Check sheet for the drawn part. Datum: minimum x, y, z corner. Units: mm. A direction names the side the tool comes from. Coordinates: 2 decimals unless noted, no trailing zeros. Write each loop counter-clockwise with the first axis right and the second up, starting at its lowest first coordinate (ties: lowest second). Pieces come first, ordered by that corner, then holes. Notation, with made-up numbers: M -9.75,65.5 L 9.25,65.5 A22 ccw 9.25,85.5 Z; hole C -17.75,-21.5 d1. An arc over 180 degrees is marked long. Answer as CSV lines item,"result". Start each with the question number.
Q1. Thickness scan on line 1 along Y through (x, z) = (11, 17.25) (3 decimals); line 2 along Z through (x, y) = (8.25, 4); line 3 along Z through (x, y) = (6.5, 9.5) (1 decimal). Record the ranges inside material, lowest first. Write a range as from..to.
Q2. Sectioned sample at B-B, the plane x = 6.5. Record the cut outline in (y, z) (1 decimal).
Q3. Sectioned sample at C-C, the plane z = 3.5. Record the cut outline in (x, y) (3 decimals).
Q4. Sectioned sample at D-D, the plane x = 3.5. Record the cut outline in (y, z) (3 decimals).
Q5. Sectioned sample at A-A, the plane y = 1.5. Record the cut outline in (x, z), then the cut area to 3 significant figures.
Q6. Access from +Z, -Z, +X, -X, +Y, -Y to the whole of each face (thin tool, end or side, straight path). Record for the marked faces 1 and 2.
Q7. Depth check by flat-ended pin: pin 1 Ø1 at (x, z) = (4.5, 6.5) entering from +Y (3 decimals); pin 2 Ø3 at (y, z) = (9.5, 13) entering from -X; pin 3 Ø4 at (x, z) = (12.5, 4) entering from -Y; pin 4 Ø1.5 at (y, z) = (9.5, 9) entering from -X. Enter the tip coordinate at first touch or a pass-through.
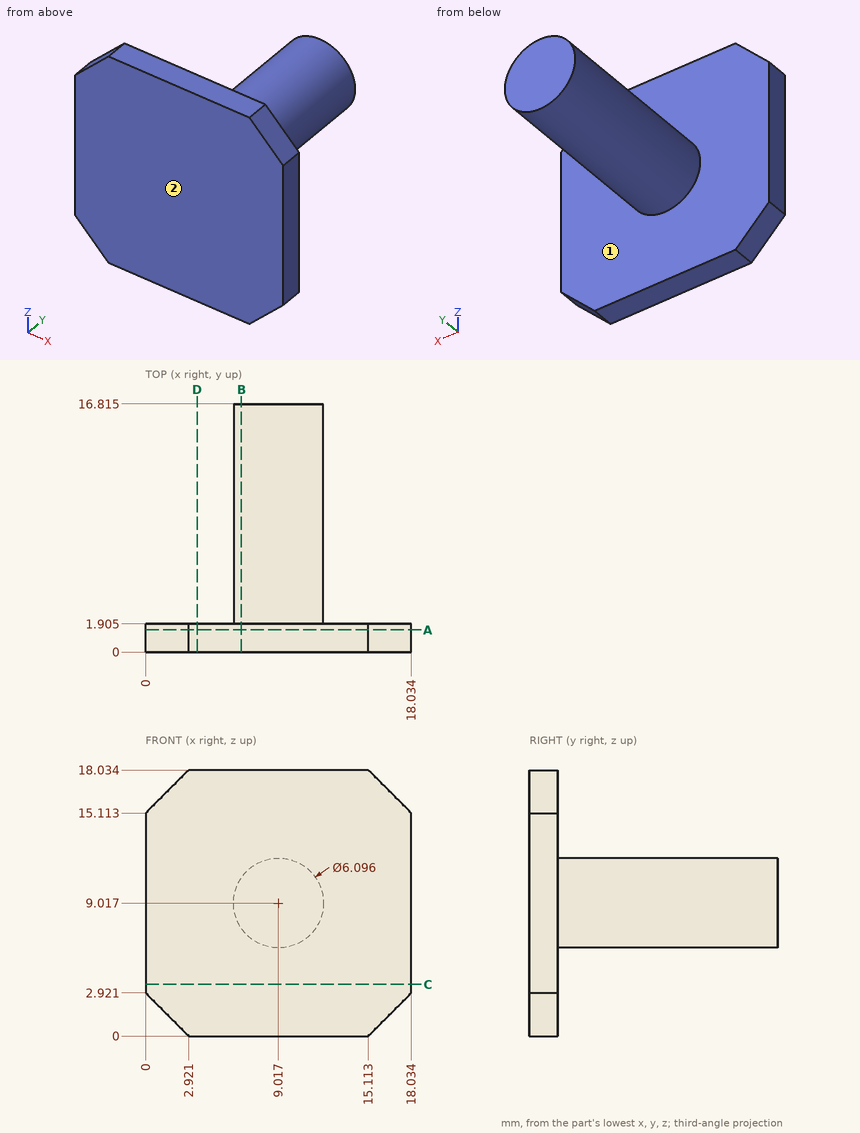
Output:
1,line 1,"y = 0..1.905"
1,line 2,"z = 6.07..11.97"
1,line 3,"z = 7.3..10.7"
2,outline,"M 0,0 L 1.9,0 L 1.9,7.3 L 16.8,7.3 L 16.8,10.7 L 1.9,10.7 L 1.9,18 L 0,18 Z"
3,outline,"M 0,0 L 18.034,0 L 18.034,1.905 L 0,1.905 Z"
4,outline,"M 0,0 L 1.905,0 L 1.905,18.034 L 0,18.034 Z"
5,outline,"M 0,2.92 L 2.92,0 L 15.11,0 L 18.03,2.92 L 18.03,15.11 L 15.11,18.03 L 2.92,18.03 L 0,15.11 Z"
5,area,"308 mm^2"
6,face 1,"+Y"
6,face 2,"+Z, -Z, +X, -X, -Y"
7,pin 1,"stops at y = 1.905"
7,pin 2,"stops at x = 7.25"
7,pin 3,"stops at y = 0"
7,pin 4,"stops at x = 5.97"
